```python
from build123d import *

# Parameters (mm, degrees)
BOSS_EXTRUDE1_DEPTH      = 20
BOSS_EXTRUDE1_2_DEPTH    = 20
SKETCH2_R                = 47
BOSS_EXTRUDE2_DEPTH      = 18
SKETCH3_R                = 45
BOSS_EXTRUDE3_DEPTH      = 2
SKETCH4_R                = 7
CUT_EXTRUDE1_DEPTH       = 1
CHAMFER1_SIZE            = 1
BOSS_EXTRUDE4_START      = 1
SKETCH5_R                = 7
BOSS_EXTRUDE4_DEPTH      = 1
BOSS_EXTRUDE5_DEPTH      = 1
BOSS_EXTRUDE6_DEPTH      = 0.1
BOSS_EXTRUDE6_DEPTH_BACK = 1


with BuildPart() as part:
    # Sketch1 → Boss-Extrude1 (new body)
    with BuildSketch(Plane.XY):
        with BuildLine():
            Line((47, 0), (49.914957884, -2.914957884))
            ThreePointArc((49.914957884, -2.914957884), (0, -50), (-49.914957884, -2.914957884))
            Line((-49.914957884, -2.914957884), (-47, 0))
            ThreePointArc((-47, 0), (0, -47), (47, 0))
        make_face()
    extrude(amount=BOSS_EXTRUDE1_DEPTH)



with BuildPart() as body_2:
    # Sketch1 → Boss-Extrude1 2 (new body)
    with BuildSketch(Plane.XY):
        with BuildLine():
            Line((50, 0), (46.913413371, 2.851604096))
            ThreePointArc((46.913413371, 2.851604096), (0.125706164, 46.999831893), (-46.89748844, 3.10251156))
            Line((-46.89748844, 3.10251156), (-50, 0))
            ThreePointArc((-50, 0), (0, 50), (50, 0))
        make_face()
    extrude(amount=BOSS_EXTRUDE1_2_DEPTH)


with BuildPart() as part_1:
    add(part.part)

    add(body_2.part)  # Boss-Extrude2 merges body 2
    # Sketch2 → Boss-Extrude2 (add)
    with BuildSketch(Plane.XY):
        Circle(SKETCH2_R)
    extrude(amount=BOSS_EXTRUDE2_DEPTH)

    # Sketch3 → Boss-Extrude3 (add)
    with BuildSketch(Plane.XY.offset(18)):
        Circle(SKETCH3_R)
    extrude(amount=BOSS_EXTRUDE3_DEPTH)

    # Sketch4 → Cut-Extrude1 (cut)
    with BuildSketch(Plane.XY.offset(20)):
        with Locations((0, -29.128438865)):
            Circle(SKETCH4_R)
    extrude(amount=-CUT_EXTRUDE1_DEPTH, mode=Mode.SUBTRACT)

    # Chamfer1
    chamfer1_edges = [part_1.edges().sort_by_distance(p)[0] for p in [
        (-7, -29.128438865, 20),
    ]]
    chamfer(chamfer1_edges, length=CHAMFER1_SIZE - 0.0001)  # a hair under: the kernel refuses the full size

    # Sketch5 → Boss-Extrude4 (add)
    with BuildSketch(Plane.XY.offset(19).offset(BOSS_EXTRUDE4_START)):
        with Locations((0, -29.128438865)):
            Circle(SKETCH5_R)
    extrude(amount=-BOSS_EXTRUDE4_DEPTH)

    # Sketch7 → Boss-Extrude5 (add)
    with BuildSketch(Plane.XY.offset(20)):
        with BuildLine():
            Line((14.249883761, 42.684198631), (14.249883761, 19.069697386))
            ThreePointArc((14.249883761, 19.069697386), (0, 4.819813625), (-14.249883761, 19.069697386))
            Line((-14.249883761, 19.069697386), (-14.249883761, 42.684198631))
            ThreePointArc((-14.249883761, 42.684198631), (0, 45), (14.249883761, 42.684198631))
        make_face()
    extrude(amount=BOSS_EXTRUDE5_DEPTH)

    # Sketch8 → Boss-Extrude6 (add, two sides: drawn at the far end of the back side and taken through both)
    with BuildSketch(Plane.XY.offset(21).offset(-BOSS_EXTRUDE6_DEPTH_BACK)):
        with BuildLine():
            Line((18.72043553, 40.921208359), (18.72043553, 20.466744814))
            ThreePointArc((18.72043553, 20.466744814), (0, 1.746309284), (-18.72043553, 20.466744814))
            Line((-18.72043553, 20.466744814), (-18.72043553, 40.921208359))
            ThreePointArc((-18.72043553, 40.921208359), (-18.1632897, 41.1715303), (-17.602797587, 41.414267072))
            Line((-17.602797587, 41.414267072), (-17.602797587, 20.466744814))
            ThreePointArc((-17.602797587, 20.466744814), (0, 2.863947227), (17.602797587, 20.466744814))
            Line((17.602797587, 20.466744814), (17.602797587, 41.414267072))
            ThreePointArc((17.602797587, 41.414267072), (18.1632897, 41.1715303), (18.72043553, 40.921208359))
        make_face()
    extrude(amount=BOSS_EXTRUDE6_DEPTH + BOSS_EXTRUDE6_DEPTH_BACK)


solid = part_1.part
```
Check sheet for the modelled part. Datum: model origin and axes. Units: mm. A direction names the side the tool comes from. Round coordinates to 2 decimals unless told otherwise and drop trailing zeros. Order: outer loops, then holes, each group sorted by start corner. A loop starts at its lowest first (then second) coordinate and runs counter-clockwise, first axis right, second up.
1) Section check D-D (x = 31.5). Record the boundary of the cut face in (y, z), and give its area (3 significant figures).
2) Section check A-A (x = 0). Record the boundary of the cut face in (y, z), and give its area (3 significant figures).
3) Mould release check, pull along Y, two halves, no side actions. Record for faces 1 (the flat face through (0.1, 2.6, 21.1)), 2 (the flat face through (45.04, -3.26, 18)), 3 (the cylindrical face through (0.41, 1.75, 20.54)), 4 (the cylindrical face through (-1.099, 49.988, 9.86)): +Y half, -Y half, draft (parallel to the pull), parting line (faces both ways), or undercut.
4) Scan lines: line 1 (Z direction, x = 3, y = -39); line 2 (X direction, y = -12.5, z = 19.25); line 3 (Y direction, x = -17.5, z = 5). Record each from-to range of solid material in increasing order.
5) Tool access check on faces 5 (the cylindrical face through (1.117, 46.987, 18.986)), 6 (the flat face through (0.2, 47.3, 20)), 7 (the flat face through (0, -29, 20)), 8 (the cylindrical face through (1.06, -49.99, 9.86)). Record the directions out of +Z, -Z, +X, -X, +Y, -Y that give a thin tool (end or side, any length) a straight path to the whole face; none if there is none.
6) Section check C-C (y = 12.5). Record the boundary of the cut face in (x, z), and give its area (3 significant figures).
7) Go/stop test with flat-tipped pins: pin 1 Ø0.9 at (y, z) = (33, 20.5) entering from -X; pin 2 Ø5 at (x, z) = (-14, 14) entering from +Y; pin 3 Ø12 at (y, z) = (38, 5.5) entering from -X; pin 4 Ø23 at (x, y) = (-5, 16.5) entering from +Z. Record where each tip stops, or that it passes through.
8) Section check B-B (z = 10.5). Record the boundary of the cut face in (x, y), and give its area (3 significant figures).
Result:
1. outline: (-38.83, 0) - (38.83, 0) - (38.83, 20) - (34.88, 20) - (34.88, 18) - (32.14, 18) - (32.14, 20) - (-32.14, 20) - (-32.14, 18) - (-34.88, 18) - (-34.88, 20) - (-38.83, 20) - close
1. area: 1,540 mm2
2. outline: (-50, 0) - (50, 0) - (50, 20) - (47, 20) - (47, 18) - (45, 18) - (45, 21) - (4.82, 21) - (4.82, 20) - (2.86, 20) - (2.86, 21.1) - (1.75, 21.1) - (1.75, 20) - (-21.13, 20) - (-22.13, 19) - (-22.13, 20) - (-36.13, 20) - (-36.13, 19) - (-37.13, 20) - (-45, 20) - (-45, 18) - (-47, 18) - (-47, 20) - (-50, 20) - close
2. area: 2,030 mm2
3. face 1: draft
3. face 2: undercut
3. face 3: -Y half
3. face 4: +Y half
4. line 1: z = 0 to 20
4. line 2: x = -48.41 to -45.31, -43.23 to 43.23, 45.31 to 48.41
4. line 3: y = -46.84 to 46.84
5. face 5: +Z
5. face 6: +Z, +Y
5. face 7: +Z, +X, -X, -Y
5. face 8: +Z, -Z, -Y
6. outline: (-48.41, 0) - (48.41, 0) - (48.41, 20) - (45.31, 20) - (45.31, 18) - (43.23, 18) - (43.23, 20) - (16.94, 20) - (16.94, 21.1) - (15.7, 21.1) - (15.7, 20) - (12.65, 20) - (12.65, 21) - (-12.65, 21) - (-12.65, 20) - (-15.7, 20) - (-15.7, 21.1) - (-16.94, 21.1) - (-16.94, 20) - (-43.23, 20) - (-43.23, 18) - (-45.31, 18) - (-45.31, 20) - (-48.41, 20) - close
6. area: 1,960 mm2
7. pin 1: stops at x = -18.72
7. pin 2: stops at y = 48.66
7. pin 3: stops at x = -38.42
7. pin 4: stops at z = 21.1
8. outline: (-50, 0) - (-46.9, 3.1) arc R47 ccw to (-47, 0) - (-49.91, -2.91) arc R50 ccw to (49.91, -2.91) - (47, 0) arc R47 ccw to (46.91, 2.85) - (50, 0) arc R50 ccw to start
8. area: 7,840 mm2
